Check sheet for the modelled part. Datum: model origin and axes. Units: mm. A direction names the side the tool comes from. Round coordinates to 2 decimals unless told otherwise and drop trailing zeros. Write each loop counter-clockwise with the first axis right and the second up, starting at its lowest first coordinate (ties: lowest second). Pieces come first, ordered by that corner, then holes. Notation, with made-up numbers: (-13, -35) -> (42, -35) arc R34 cw to (42, 1) -> close; hole circle Ø1 at (32, 81.25). An arc over 180 degrees is marked (long way). One line per item, written item: value.
from build123d import *

# Parameters (mm, degrees)
RESSALTO_EXTRUS_O1_DEPTH      = 25
ESBO_O3_R                     = 2.25
RESSALTO_EXTRUS_O2_DEPTH      = 3
ESBO_O6_R                     = 1.25
CORTE_EXTRUS_O2_DEPTH         = 10
RESSALTO_EXTRUS_O3_DEPTH      = 5
RESSALTO_EXTRUS_O3_DEPTH_BACK = 7
CORTE_EXTRUS_O1_DEPTH         = 32.980788504
FILETE1_R                     = 3
ESBO_O9_R                     = 1.75
CORTE_EXTRUS_O3_DEPTH         = 32.199307287
RESSALTO_EXTRUS_O4_DEPTH      = 8.8
RESSALTO_EXTRUS_O5_DEPTH      = 20.2
ESBO_O14_R                    = 1.25
CORTE_EXTRUS_O4_DEPTH         = 47.082463565
FILETE2_R                     = 3
FILETE3_R                     = 3


# Some blends are built 0.0001 mm under size
with BuildPart() as part:
    # Esboço1 → Ressalto-extrusão1 (new body)
    with BuildSketch(Plane(origin=(0, 0, 0), x_dir=(1, 0, 0), z_dir=(0, 1, 0))):
        Polygon((7.25, 4.185789452), (0, 8.371578903), (-7.25, 4.185789452), (-7.25, -4.185789452), (0, -8.371578903), (7.25, -4.185789452), align=None)
    extrude(amount=RESSALTO_EXTRUS_O1_DEPTH)

    # Esboço3 → Ressalto-extrusão2 (add)
    with BuildSketch(Plane(origin=(-3.625, 0, 6.278684177), x_dir=(0.8660254037844387, 0, 0.4999999999999999), z_dir=(-0.49999999999999994, 0, 0.8660254037844388))):
        with Locations(Location((0, 7, 0), (0, 0, 180))):
            Circle(ESBO_O3_R)
        with Locations(Location((0, 18, 0), (0, 0, 180))):
            Circle(ESBO_O3_R)
    extrude(amount=RESSALTO_EXTRUS_O2_DEPTH)

    # Esboço4 → Revolução1 (revolve)
    with BuildSketch(Plane(origin=(0, 18, 0), x_dir=(1, 0, 0), z_dir=(0, 1, 0))):
        Polygon((-7.073557159, -7.751760389), (-6.872595264, -4.403684177), (-5.573557159, -5.153684177), align=None)
    revolve(axis=Axis((-2.565266445, 18, 4.443171818), (-0.5000000000000001, 0, 0.8660254037844386)))

    # Esboço5 → Revolução2 (revolve)
    with BuildSketch(Plane(origin=(0, 7, 0), x_dir=(-1, 0, 0), z_dir=(0, -1, 0)), mode=Mode.PRIVATE) as revolu_o2_sk:
        Polygon((7.073557159, -7.751760389), (5.573557159, -5.153684177), (6.872595264, -4.403684177), align=None)
    revolve(revolu_o2_sk.sketch.rotate(Axis((-5.573557159, 7, 9.653684177), (0.4999999999999998, 0, -0.8660254037844388)), 180), axis=Axis((-5.573557159, 7, 9.653684177), (0.4999999999999998, 0, -0.8660254037844388)))

    # Esboço6 → Corte-extrusão2 (cut)
    with BuildSketch(Plane(origin=(-5.125, 0, 8.876760389), x_dir=(0.8660254037844386, 0, 0.5), z_dir=(-0.5000000000000001, 0, 0.8660254037844387))):
        with Locations((0, 18)):
            Circle(ESBO_O6_R)
        with Locations(Location((0, 7, 0), (0, 0, 180))):
            Circle(ESBO_O6_R)
    extrude(amount=-CORTE_EXTRUS_O2_DEPTH, mode=Mode.SUBTRACT)

    # Esboço8 → Ressalto-extrusão3 (add, two sides: drawn at the far end of the back side and taken through both)
    with BuildSketch(Plane(origin=(3.625, 0, -6.278684177), x_dir=(-0.8660254037844386, 0, -0.4999999999999999), z_dir=(0.49999999999999994, 0, -0.8660254037844387)).offset(-RESSALTO_EXTRUS_O3_DEPTH_BACK)):
        Polygon((-4.128938216, 20.871578903), (8.371578903, 8.371061784), (4.128938216, 4.128421097), (-8.371578903, 16.628938216), align=None)
    extrude(amount=RESSALTO_EXTRUS_O3_DEPTH + RESSALTO_EXTRUS_O3_DEPTH_BACK)

    # Esboço2 → Corte-extrusão1 (cut, through all)
    with BuildSketch(Plane(origin=(0, 25, 0), x_dir=(1, 0, 0), z_dir=(0, 1, 0))):
        Polygon((0, 6.92820323), (-6, 3.464101615), (-6, -3.464101615), (0, -6.92820323), (6, -3.464101615), (6, 3.464101615), align=None)
    extrude(amount=-CORTE_EXTRUS_O1_DEPTH, mode=Mode.SUBTRACT)

    # Filete1
    filete1_edges = [part.edges().sort_by_distance(p)[0] for p in [
        (7.962117307, 10.378679656, -9.548151025),
        (4.287882693, 14.621320344, -11.669471368),
    ]]
    fillet(filete1_edges, radius=FILETE1_R - 0.0001)  # a hair under: the kernel refuses the full size

    # Esboço9 → Corte-extrusão3 (cut, through all)
    with BuildSketch(Plane(origin=(-0.000223919, -0.00025856, -0.00012928), x_dir=(0.7905694150420967, -0.547722557505165, -0.27386127875258026), z_dir=(-0.6123724356957922, -0.7071067811865502, -0.3535533905932724))):
        with Locations(Location((-0.996318298, -12.755189134, 0), (0, 0, 17.023866185))):
            Circle(ESBO_O9_R)
    extrude(amount=-CORTE_EXTRUS_O3_DEPTH, mode=Mode.SUBTRACT)

    # Esboço10 → Ressalto-extrusão4 (add)
    with BuildSketch(Plane(origin=(-7.249776081, 8.371320344, -4.185660172), x_dir=(0.7905694150420924, 0.5477225575051679, -0.2738612787525866), z_dir=(-0.6123724356957977, 0.707106781186544, -0.3535533905932755))):
        Polygon((5.849930433, 7.165250453), (4.585019369, 5.616057115), (18.278649783, -5.564745298), (19.543560847, -4.01555196), align=None)
    extrude(amount=RESSALTO_EXTRUS_O4_DEPTH)

    # Esboço13 → Ressalto-extrusão5 (add)
    with BuildSketch(Plane(origin=(-12.638653515, 14.593860018, -7.296930009), x_dir=(0.7905694150420924, 0.547722557505168, -0.27386127875258653), z_dir=(-0.6123724356957978, 0.707106781186544, -0.35355339059327534))):
        Polygon((4.585019369, 5.616057115), (5.849930433, 7.165250453), (12.69674564, 1.574849247), (11.410886615, 0), align=None)
    extrude(amount=RESSALTO_EXTRUS_O5_DEPTH)

    # Esboço14 → Corte-extrusão4 (cut, through all)
    with BuildSketch(Plane(origin=(3.641584315, 0.01920948, -6.268990093), x_dir=(0.8646985820812304, -0.0015391164783120645, 0.5022887548683287), z_dir=(-0.5022911129481685, -0.002649602595281497, 0.8646945226259835))):
        with Locations(Location((-23.342145929, 29.472416585, 0), (0, 0, 0.088185223))):
            Circle(ESBO_O14_R)
    extrude(amount=-CORTE_EXTRUS_O4_DEPTH, mode=Mode.SUBTRACT)

    # Filete2
    filete2_edges = [part.edges().sort_by_distance(p)[0] for p in [
        (-15.479198351, 35.127416998, -18.444075991),
        (-20.883800635, 28.877158438, -21.58354736),
    ]]
    fillet(filete2_edges, radius=FILETE2_R)

    # Filete3
    # the kernel refuses this fillet: 3 mm, written as the material it takes off along each edge
    with BuildSketch(Plane(origin=(1.811887952, 27.094118578, -7.325484907), x_dir=(0.6123724356957967, -0.707106781186545, 0.3535533905932749), z_dir=(0.49999999999999784, -2.3869795029440866e-15, -0.86602540378444))) as filete3_piece_1:
        with BuildLine():
            CenterArc((FILETE3_R, FILETE3_R), FILETE3_R, 180, 90)
            Line((0, FILETE3_R), (0, 0))
            Line((0, 0), (FILETE3_R, 0))
        make_face()
    extrude(amount=9.5, mode=Mode.SUBTRACT)


solid = part.part
Item 1: Release check for a two-part mould opening along X. For faces 1 (the flat face through (-3.98, 9.56, -7.47)), 2 (the cylindrical face through (-17.122, 29.585, -19.392)), 3 (the cylindrical face through (7.058, 11.104, -9.082)) record: pulls with the +X half, pulls with the -X half, needs draft (parallel to the pull), parting line crosses it, or undercut.
Result set:
face 1: pulls with the -X half
face 2: undercut
face 3: pulls with the +X half
Item 2: Material ranges on line 1 along X through (y, z) = (17.5, 4); line 2 along X through (y, z) = (15.5, -5.5); line 3 along X through (y, z) = (21.5, -4.5), recorded low to high.
Result set:
line 1: -7.25 to -5.07, 5.07 to 7.25
line 2: -4.97 to -2.47, 2.47 to 5.68, 9.47 to 11.19
line 3: -6.71 to -4.21, 4.21 to 6.71
Item 3: Sectioned sample at B-B (x = -5). State how many separate pieces and enclosed holes the cut face has, then the cut area to 3 significant figures.
Result set:
separate pieces: 3
enclosed holes: 0
area: 133 mm^2
Item 4: Tool access check on faces 4 (the flat face through (-3.57, 12.32, -6.31)), 5 (the flat face through (-2.96, 12.68, -5.22)), 6 (the flat face through (4.481, 4.752, -5.784)), 7 (the cylindrical face through (-15.515, 33.885, -18.448)). Record the directions out of +Z, -Z, +X, -X, +Y, -Y that give a thin tool (end or side, any length) a straight path to the whole face; none if there is none.
Result set:
face 4: -X
face 5: +Y, -Y
face 6: +X, -Y
face 7: +Y
Item 5: Sectioned sample at A-A (z = -14.5). Enter the section's corners in (x, y).
Result set:
outline: (-10.68, 29) -> (-10.61, 16.44) -> (-6.61, 12.98) -> (-6.61, 25.48) -> close
Item 6: Depth check by flat-ended pin: pin 1 (1 mm diameter, centred on x = -6.5, z = 6.5, fed in from +Y); pin 2 (2.5 mm diameter, centred on y = 16.5, z = 0.5, fed in from -X); pin 3 (7 mm diameter, centred on x = -0.5, z = -3, fed in from +Y). Enter the tip coordinate at first touch or a pass-through.
Result set:
pin 1: y = 20.37
pin 2: x = -7.25
pin 3: y = 25
